from build123d import *

# Parameters (mm, degrees)
SKETCH1_W           = 32.2
SKETCH1_H           = 23.5
BOSS_EXTRUDE1_DEPTH = 32.1
SKETCH2_R           = 1.5
SKETCH2_W           = 22.6
SKETCH2_H           = 12
CUT_EXTRUDE1_DEPTH  = 32.1
SKETCH3_R           = 1.5
CUT_EXTRUDE2_DEPTH  = 36.1


with BuildPart() as part:
    # Sketch1 → Boss-Extrude1 (new body)
    with BuildSketch(Plane(origin=(0, 0, 0), x_dir=(1, 0, 0), z_dir=(0, 1, 0))):
        with Locations((5.231046931, -2.217870036)):
            Rectangle(SKETCH1_W, SKETCH1_H)
    extrude(amount=BOSS_EXTRUDE1_DEPTH)

    # Sketch2 → Cut-Extrude1 (cut)
    with BuildSketch(Plane(origin=(0, 0, -9.532129964), x_dir=(-1, 0, 0), z_dir=(0, 0, -1))):
        with Locations((8.568953069, 26.1)):
            Circle(SKETCH2_R)
        with Locations((-19.031046931, 26.1)):
            Circle(SKETCH2_R)
        with Locations((-5.231046931, 5)):
            Circle(SKETCH2_R)
        with Locations((-5.231046931, 26.1)):
            Rectangle(SKETCH2_W, SKETCH2_H)
    extrude(amount=-CUT_EXTRUDE1_DEPTH, mode=Mode.SUBTRACT)

    # Sketch3 → Cut-Extrude2 (cut)
    with BuildSketch(Plane.ZY.offset(10.868953069)):
        with Locations((2.217870036, 5)):
            Circle(SKETCH3_R)
    extrude(amount=-CUT_EXTRUDE2_DEPTH, mode=Mode.SUBTRACT)


solid = part.part
The model under review builds one solid part; all positions refer to its coordinate system, in mm. A direction names the side the tool comes from. Round coordinates to 2 decimals unless told otherwise and drop trailing zeros. Write each loop counter-clockwise with the first axis right and the second up, starting at its lowest first coordinate (ties: lowest second). Pieces come first, ordered by that corner, then holes. Notation, with made-up numbers: (64.5, 72) - (90.5, 72) arc R20 cw to (90.5, 79) - close; hole circle Ø5 at (44, -37). An arc over 180 degrees is marked (long way). One line per item, written item: value. Start each with the question number.
1. Consider section A-A on y = 26.1. Write out the cut boundary in (x, z).
2. To check wall thickness, follow L1, parallel to X at y = 28, z = -3.25; L2, parallel to X at y = 5, z = -0.5; L3, parallel to Z at x = 1, y = 5. State the ranges of each line that lie inside material, in increasing order. Write a range as from..to.
3. Consider section B-B on x = -8. Write out the cut boundary in (y, z).
4. Consider section D-D on z = 6.25. Write out the cut boundary in (x, y), and give its area (3 significant figures).
5. The part is to be moulded in two halves that separate along Z. For faces 3 (the face through (13.17, 3.67, 2.91)), 4 (the face through (19, 32.1, 2)), 5 (the face through (5, 12, -9.532)), 6 (the face through (-2.932, 4.425, 3.603)), say which applies: released by +Z, released by -Z, zero draft, split by the parting line, or undercut.
6. Machinability: for faces 1 (the face through (-6.069, 26, 2)), 2 (the face through (5.556, 3.536, -3.739)), which of the approach directions +Z, -Z, +X, -X, +Y, -Y give a long, thin tool a straight path to every point of the face, cutting with its end or side? Answer none if there is none.
7. Clearance check with a flat-ended pin moving along its axis: P1, Ø6, axis at x = 10.5, z = -3, coming from the +Y side. State where the tip first meets the part, or that it passes through.
8. Consider section C-C on y = 22.5. Write out the cut boundary in (x, z).
Checks:
1. outline: (-10.87, -9.53) - (-10.07, -9.53) - (-10.07, 13.97) - (-10.87, 13.97) - close; (-7.07, -9.53) - (-6.07, -9.53) - (-6.07, 13.97) - (-7.07, 13.97) - close; (16.53, -9.53) - (17.53, -9.53) - (17.53, 13.97) - (16.53, 13.97) - close; (20.53, -9.53) - (21.33, -9.53) - (21.33, 13.97) - (20.53, 13.97) - close
2. L1: x = -10.87..-6.07, 16.53..21.33
2. L2: x = -10.87..3.73, 6.73..21.33
2. L3: z = -9.53..0.72, 3.72..13.97
3. outline: (0, -9.53) - (24.71, -9.53) - (24.71, 13.97) - (0, 13.97) - close; (27.49, -9.53) - (32.1, -9.53) - (32.1, 13.97) - (27.49, 13.97) - close; hole circle Ø3 at (5, 2.22)
4. outline: (-10.87, 0) - (21.33, 0) - (21.33, 32.1) - (16.53, 32.1) - (16.53, 20.1) - (-6.07, 20.1) - (-6.07, 32.1) - (-10.87, 32.1) - close; hole circle Ø3 at (-8.57, 26.1); hole circle Ø3 at (5.23, 5); hole circle Ø3 at (19.03, 26.1)
4. area: 741 mm^2
5. face 3: undercut
5. face 4: zero draft
5. face 5: released by -Z
5. face 6: undercut
6. face 1: +Z, -Z, +Y
6. face 2: +Z, -Z
7. P1: stops at y = 20.1
8. outline: (-10.87, -9.53) - (-6.07, -9.53) - (-6.07, 13.97) - (-10.87, 13.97) - close; (16.53, -9.53) - (21.33, -9.53) - (21.33, 13.97) - (16.53, 13.97) - close
